from build123d import *
from build123d import SkipClean  # not in build123d's __all__

# Parameters (mm, degrees)
F0_R      = 28.575
F2_R      = 11.1125
F4_R      = 7.9375
F5_DEPTH  = 50.8010001
F6_R      = 28.575
F6_R_2    = 7.9375
F7_DEPTH  = 15.875
F10_DEPTH = 9.525
F11_W     = 38.1
F11_H     = 85.725
F12_DEPTH = 9.525
F13_R     = 6.746875
F14_DEPTH = 9.526


# Not quite as in the source:
# - after a boolean that leaves OpenCascade's solid faulty, fix() repairs it


with BuildPart() as f3:
    # F0 (on Front) → F3 section 0
    with BuildSketch(Plane.XZ):
        Circle(F0_R)
    # F2 (on offset) → F3 section 1
    with BuildSketch(Plane.XZ.offset(50.8)):
        Circle(F2_R)
    loft()

    # F4 (on face) → F5 (cut, through all)
    with BuildSketch(Plane.XZ.offset(50.8)):
        Circle(F4_R)
    extrude(amount=-F5_DEPTH, mode=Mode.SUBTRACT)

    # F6 (on face) → F7 (join)
    with BuildSketch(Plane(origin=(0, 0, 0), x_dir=(-1, 0, 0), z_dir=(0, 1, 0))):
        Circle(F6_R)
        Circle(F6_R_2, mode=Mode.SUBTRACT)
    with SkipClean():  # cleaning this boolean's faces spoils the solid; the shape is the same uncleaned
        extrude(amount=F7_DEPTH)

    # F9 (on offset) → F10 (join)
    with BuildSketch(Plane.XZ.offset(-3.175)):
        with BuildLine():
            ThreePointArc((19.05, -21.2985474857), (0, -28.575), (-19.05, -21.2985474857))
            Line((-19.05, -21.2985474857), (-19.05, -152.4))
            Line((-19.05, -152.4), (19.05, -152.4))
            Line((19.05, -152.4), (19.05, -21.2985474857))
        make_face()
    extrude(amount=-F10_DEPTH)

    add(f3.part.fix(), mode=Mode.REPLACE)

    # F11 (on face) → F12 (join)
    with BuildSketch(Plane(origin=(0, 0, -152.4), x_dir=(1, 0, 0), z_dir=(0, 0, -1))):
        with Locations((0, -7.9375)):
            Rectangle(F11_W, F11_H)
    extrude(amount=F12_DEPTH)

    add(f3.part.fix(), mode=Mode.REPLACE)

    # F13 (on face) → F14 (cut, through all)
    with BuildSketch(Plane.XY.offset(-152.4)):
        with Locations((0, 31.75)):
            Circle(F13_R)
        with Locations((0, -15.875)):
            Circle(F13_R)
    extrude(amount=-F14_DEPTH, mode=Mode.SUBTRACT)


solid = f3.part
For this review, take the finished solid that the model builds, in its own axes (mm). A direction names the side the tool comes from. Round coordinates to 2 decimals unless told otherwise and drop trailing zeros. Loops run counter-clockwise (first coordinate to the right, second up) from the corner with the lowest first, then second, coordinate; pieces in that order, holes last. Notation, with made-up numbers: (9, -37.75) - (33, -37.75) arc R16 cw to (33, -26.75) - close; hole circle Ø7 at (-37, -16.75). An arc over 180 degrees is marked (long way). Put each result on its own line as item: value. Start each with the question number.
1. Consider section A-A on x = 0. State the section outline as (y, z) points (1 decimal), plus the area to 3 significant figures.
2. For probe 1 along Y at (x, z) = (0, -158) (3 decimals); probe 2 along Z at (x, y) = (0, 6) (1 decimal); probe 3 along X at (y, z) = (31, -155), list the stretches that pass through material, from the lowest coordinate up. Write a range as [from, to].
3. Mouldability with a two-part tool opening along Z and no side actions: class faces 6 (the flat face through (0, 12.7, -86)), 7 (the flat face through (0, 7, -161.925)), 8 (the cylindrical face through (-0.878, -9.186, -157.096)) as +Z half, -Z half, draft (parallel to the pull), parting line (faces both ways), or undercut.
4. For faces 1 (the flat face through (0, -8, -152.4)), 2 (the flat face through (-19.05, 8, -112)), 3 (the flat face through (0, -34.925, -157)), 4 (the flat face through (19.05, 8, -112)), 5 (the flat face through (-6, 15.875, -6)), list the 3-axis set-ups (+Z, -Z, +X, -X, +Y, -Y) from which the entire face can be reached by the end or side of a thin tool; tool diameter is ignored.
5. Insertion check: P1, Ø11.5, axis at x = 1.5, z = -64.5, coming from the -Y side (3 decimals); P2, Ø15.5, axis at x = 0, y = 31.75, coming from the +Z side; P3, Ø8, axis at x = 0, y = -15.875, coming from the +Z side. Each pin has a flat end and moves straight along its axis. Give the tip position at first contact, or say it passes through.
6. Consider section D-D on z = -55.5. State the section outline as (x, y) points (3 decimals), plus the area to 3 significant figures.
7. Consider section B-B on y = 31.75. State the section outline as (x, z) points (3 decimals).
8. Consider section C-C on y = -18.5. State how many separate pieces and enclosed holes the cut face has, plus the area to 3 significant figures.
Result sheet:
1. outline: (-50.8, -11.1) - (0, -28.6) - (3.2, -28.6) - (3.2, -152.4) - (-9.1, -152.4) - (-9.1, -161.9) - (25, -161.9) - (25, -152.4) - (12.7, -152.4) - (12.7, -28.6) - (15.9, -28.6) - (15.9, -7.9) - (-50.8, -7.9) - close; (-50.8, 7.9) - (15.9, 7.9) - (15.9, 28.6) - (0, 28.6) - (-50.8, 11.1) - close; (-34.9, -161.9) - (-22.6, -161.9) - (-22.6, -152.4) - (-34.9, -152.4) - close; (38.5, -161.9) - (50.8, -161.9) - (50.8, -152.4) - (38.5, -152.4) - close
1. area: 3,600 mm^2
2. probe 1: [-34.925, -22.622], [-9.128, 25.003], [38.497, 50.8]
2. probe 2: [-161.9, -7.9], [7.9, 28.6]
2. probe 3: [-19.05, -6.71], [6.71, 19.05]
3. face 6: undercut
3. face 7: -Z half
3. face 8: draft
4. face 1: +X, -X, -Y
4. face 2: -Z, -X, +Y, -Y
4. face 3: -Z, +X, -X, -Y
4. face 4: -Z, +X, +Y, -Y
4. face 5: +Z, +X, -X, +Y
5. P1: y = 3.175
5. P2: z = -152.4
5. P3: z = 24.49
6. outline: (-19.05, 3.175) - (19.05, 3.175) - (19.05, 12.7) - (-19.05, 12.7) - close
6. area: 363 mm^2
7. outline: (-19.05, -161.925) - (-6.747, -161.925) - (-6.747, -152.4) - (-19.05, -152.4) - close; (6.747, -161.925) - (19.05, -161.925) - (19.05, -152.4) - (6.747, -152.4) - close
8. separate pieces: 3
8. enclosed holes: 1
8. area: 1,600 mm^2
